Geometry check sheet. Reference: drawing and pictorial views, mm from the part's lowest x, y, z. A direction names the side the tool comes from. Give positions to 0.01 mm unless a question says otherwise; leave off trailing zeros. Order: outer loops, then holes, each group sorted by start corner. A loop starts at its lowest first (then second) coordinate and runs counter-clockwise, first axis right, second up.
Item 1: Sectioned sample at C-C on y = 3.5. Record the boundary of the cut face in (x, z).
Item 2: Material ranges on line 1 along Z through (x, y) = (2.8, 4.25); line 2 along Y through (x, z) = (3.05, 2.8); line 3 along Y through (x, z) = (4.4, 2), recorded low to high.
Item 3: Release check for a two-part mould opening along X. For the marked faces 1, 2 and 3 record: released by +X, released by -X, zero draft, split by the parting line, or undercut.
Item 4: Gauge pin test, flat ends, axial feed: P1, Ø1.5, axis at x = 5, z = 4.5, coming from the -Y side; P2, Ø3, axis at y = 4, z = 4.5, coming from the -X side; P3, Ø2, axis at x = 5, y = 2.5, coming from the +Z side; P4, Ø1, axis at y = 4.5, z = 3.5, coming from the +X side. Record the tip position at first contact, or that the pin passes through.
Item 5: Sectioned sample at A-A on x = 2.85. Record the boundary of the cut face in (y, z).
Item 6: Sectioned sample at B-B on y = 2.25. Record the boundary of the cut face in (x, z).
Item 7: Access from +Z, -Z, +X, -X, +Y, -Y to the whole of each face (thin tool, end or side, straight path). Record for the marked faces 4 and 5.
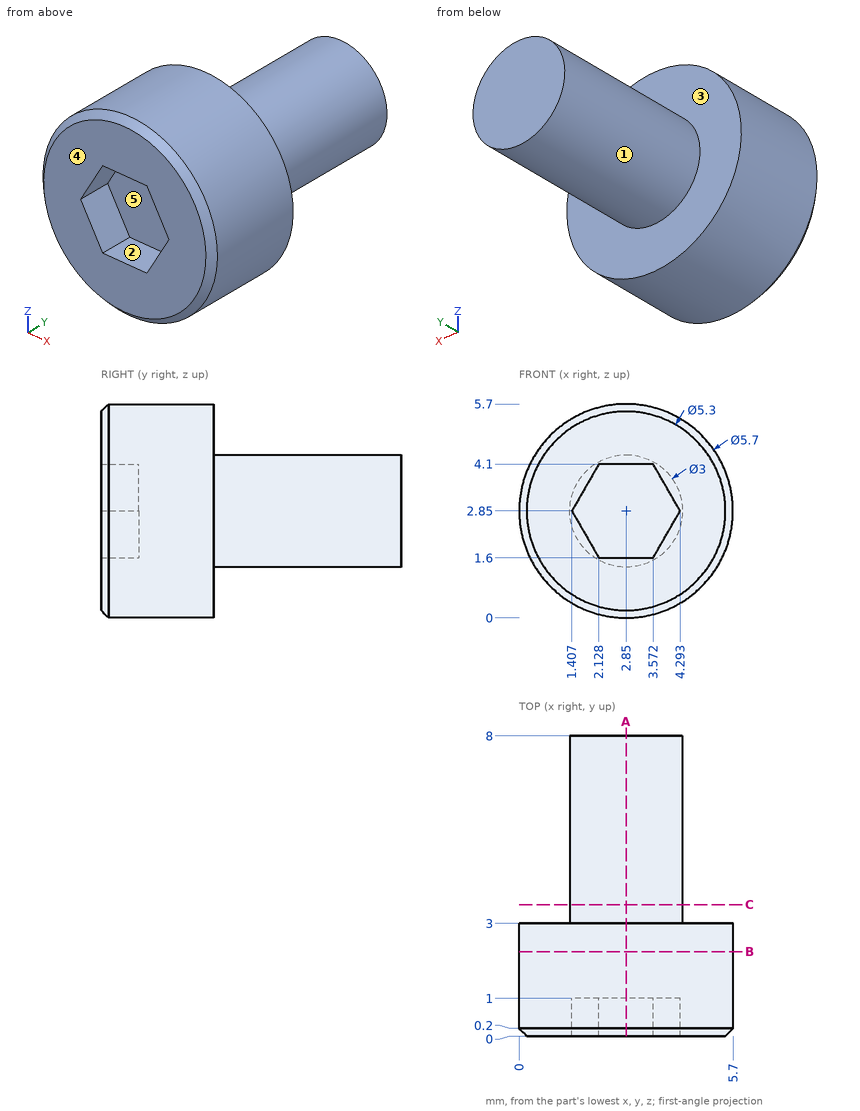
Report:
1. outline: circle Ø3 at (2.85, 2.85)
2. line 1: z = 1.35 to 4.35
2. line 2: y = 1 to 8
2. line 3: y = 0 to 3
3. face 1: split by the parting line
3. face 2: undercut
3. face 3: zero draft
4. P1: stops at y = 0
4. P2: stops at x = 0.05
4. P3: stops at z = 5.46
4. P4: stops at x = 4.34
5. outline: (0, 0.2) - (0.2, 0) - (3, 0) - (3, 1.35) - (8, 1.35) - (8, 4.35) - (3, 4.35) - (3, 5.7) - (0.2, 5.7) - (0, 5.5) - (0, 4.1) - (1, 4.1) - (1, 1.6) - (0, 1.6) - close
6. outline: circle Ø5.7 at (2.85, 2.85)
7. face 4: +Z, -Z, +X, -X, -Y
7. face 5: -Y
